```python
from build123d import *

# Parameters (mm, degrees)
SKETCH1_R           = 1.275
BOSS_EXTRUDE1_DEPTH = 5
SKETCH2_W           = 9.1
SKETCH2_H           = 17.8
BOSS_EXTRUDE2_DEPTH = 25
BOSS_EXTRUDE3_DEPTH = 3
CUT_EXTRUDE1_DEPTH  = 15


with BuildPart() as part:
    # Sketch1 → Boss-Extrude1 (new body)
    # profile 1 of 2: a face of its own
    with BuildSketch(Plane(origin=(0, 0, 0), x_dir=(0, 0, -1), z_dir=(1, 0, 0))):
        Polygon((-4.381647728, -34.17856484), (-0.382647728, -30.17956484), (-0.382647728, 8.02143516), (-6.482647728, 8.02143516), (-9.382647728, 8.02143516), (-9.382647728, -34.17856484), align=None)
        with Locations((-5.982647728, 2.42143516)):
            Circle(SKETCH1_R, mode=Mode.SUBTRACT)
        with Locations((-5.982647728, -28.57856484)):
            Circle(SKETCH1_R, mode=Mode.SUBTRACT)
    # profile 2 of 2: a face of its own
    with BuildSketch(Plane(origin=(0, 0, 0), x_dir=(0, 0, -1), z_dir=(1, 0, 0))):
        Polygon((2.617352272, 8.02143516), (2.617352272, 25.82143516), (-6.482647728, 25.82143516), (-6.482647728, 8.02143516), (-0.382647728, 8.02143516), align=None)
    extrude(amount=BOSS_EXTRUDE1_DEPTH)

    # Sketch2 → Boss-Extrude2 (add)
    with BuildSketch(Plane(origin=(5, 0, 0), x_dir=(0, 0, -1), z_dir=(1, 0, 0))):
        with Locations((-1.932647728, 16.92143516)):
            Rectangle(SKETCH2_W, SKETCH2_H)
    extrude(amount=BOSS_EXTRUDE2_DEPTH)

    # Sketch3 → Boss-Extrude3 (add)
    with BuildSketch(Plane(origin=(0, 0, 0.382647728), x_dir=(-1, 0, 0), z_dir=(0, 0, -1))):
        Polygon((-30, 8.02143516), (0, 8.02143516), (0, -30.17956484), (-5, -30.17956484), align=None)
    extrude(amount=BOSS_EXTRUDE3_DEPTH)

    # Sketch4 → Cut-Extrude1 (cut, symmetric)
    with BuildSketch(Plane(origin=(5, 0, 0), x_dir=(0, 0, -1), z_dir=(1, 0, 0))):
        Polygon((-0.382647728, -30.17956484), (2.617352272, -27.17956484), (2.617352272, -30.17956484), align=None)
    extrude(amount=CUT_EXTRUDE1_DEPTH, both=True, mode=Mode.SUBTRACT)


solid = part.part
```
The model under review builds one solid part; all positions refer to its coordinate system, in mm. A direction names the side the tool comes from. Round coordinates to 2 decimals unless told otherwise and drop trailing zeros. Loops run counter-clockwise (first coordinate to the right, second up) from the corner with the lowest first, then second, coordinate; pieces in that order, holes last.
Item 1: For line 1 (Y direction, x = 10.25, z = 2.5); line 2 (Y direction, x = 24.75, z = -0.5); line 3 (X direction, y = -25, z = 6.5), list the stretches that pass through material, from the lowest coordinate up.
Determined:
line 1: y = 8.02 to 25.82
line 2: y = 0 to 25.82
line 3: x = 0 to 5
Item 2: Take a section at D-D (x = 5.75). Write out the cut boundary in (y, z), then the cut area to 3 significant figures.
Determined:
outline: (-29.03, -0.76) - (-27.18, -2.62) - (25.82, -2.62) - (25.82, 6.48) - (8.02, 6.48) - (8.02, 0.38) - (-29.03, 0.38) - close
area: 271 mm2
Item 3: Take a section at C-C (y = 19). Write out the cut boundary in (x, z).
Determined:
outline: (0, -2.62) - (30, -2.62) - (30, 6.48) - (0, 6.48) - close
Item 4: Take a section at B-B (z = 3.25). Write out the cut boundary in (x, y), then the cut area to 3 significant figures.
Determined:
outline: (0, -33.05) - (5, -33.05) - (5, 8.02) - (30, 8.02) - (30, 25.82) - (0, 25.82) - close
area: 739 mm2
Item 5: Mouldability with a two-part tool opening along Y and no side actions: class faces 4 (the face through (2.465, 2.804, 4.767)), 5 (the face through (2.465, -29.823, 6.259)), 6 (the face through (30, 17, 2)), 7 (the face through (2, -34.179, 7)) as released by +Y, released by -Y, zero draft, split by the parting line, or undercut.
Determined:
face 4: undercut
face 5: undercut
face 6: zero draft
face 7: released by -Y
Item 6: Clearance check with flat-ended pins moving along their axes: pin 1 Ø3 at (y, z) = (9, 1) entering from -X; pin 2 Ø3.5 at (y, z) = (2.42, 5.98) entering from +X; pin 3 Ø6 at (x, z) = (10, -0.5) entering from -Y; pin 4 Ø10 at (x, y) = (21.5, 1.5) entering from +Z. State where each tip first meets the part, or that it passes through.
Determined:
pin 1: stops at x = 0
pin 2: stops at x = 5
pin 3: stops at y = -27.12
pin 4: stops at z = 0.38
Item 7: For faces 1 (the face through (2, 8.021, 8)), 2 (the face through (17, 8.021, 3)), 3 (the face through (2.757, -30.728, 0.931)), list the 3-axis set-ups (+Z, -Z, +X, -X, +Y, -Y) from which the entire face can be reached by the end or side of a thin tool; tool diameter is ignored.
Determined:
face 1: +Z, +X, -X, +Y
face 2: +Z, +X, -Y
face 3: -Z, +X, -X, -Y
Item 8: Take a section at A-A (x = 23). Write out the cut boundary in (y, z), then the cut area to 3 significant figures.
Determined:
outline: (-2.67, -2.62) - (25.82, -2.62) - (25.82, 6.48) - (8.02, 6.48) - (8.02, 0.38) - (-2.67, 0.38) - close
area: 194 mm2
